from build123d import *

# Parameters (mm, degrees)
EXTRUDE_1_DEPTH     = 26
SKETCH_2_R          = 3.5
SKETCH_2_R_2        = 1.6
SKETCH_2_R_3        = 2
CUT_EXTRUDE_2_DEPTH = 155.518607294
CUT_EXTRUDE_5_DEPTH = 155.518607294
SKETCH_5_R          = 10.5
CUT_EXTRUDE_6_DEPTH = 1.6
CUT_EXTRUDE_START   = -1.6
SKETCH_6_R          = 10.5
CUT_EXTRUDE_7_DEPTH = 1.6
SKETCH_7_R          = 10.5
CUT_EXTRUDE_8_DEPTH = 1.6
SKETCH_8_R          = 10.5
CUT_EXTRUDE_9_DEPTH = 1.6


with BuildPart() as part:
    # 草图1 → 凸台-拉伸1 (new body)
    with BuildSketch(Plane(origin=(0, 0, 0), x_dir=(1, 0, 0), z_dir=(0, 1, 0))):
        with BuildLine():
            Line((0, 0), (0, 140))
            Line((0, 140), (5, 140))
            Line((5, 140), (5, 85))
            ThreePointArc((5, 85), (7.928932188, 77.928932188), (15, 75))
            Line((15, 75), (45, 75))
            ThreePointArc((45, 75), (52.071067812, 77.928932188), (55, 85))
            Line((55, 85), (55, 140))
            Line((55, 140), (60, 140))
            Line((60, 140), (60, 0))
            Line((60, 0), (55, 0))
            Line((55, 0), (55, 55))
            ThreePointArc((55, 55), (52.071067812, 62.071067812), (45, 65))
            Line((45, 65), (15, 65))
            ThreePointArc((15, 65), (7.928932188, 62.071067812), (5, 55))
            Line((5, 55), (5, 0))
            Line((5, 0), (0, 0))
        make_face()
    extrude(amount=EXTRUDE_1_DEPTH)

    # 草图2 → 切除-拉伸2 (cut, through all)
    with BuildSketch(Plane(origin=(60, 0, 0), x_dir=(0, 0, -1), z_dir=(1, 0, 0))):
        with Locations((128, 13)):
            Circle(SKETCH_2_R)
        with Locations((123, 18)):
            Circle(SKETCH_2_R_2)
        with Locations((133, 18)):
            Circle(SKETCH_2_R_2)
        with Locations((133, 8)):
            Circle(SKETCH_2_R_2)
        with Locations((123, 8)):
            Circle(SKETCH_2_R_2)
        with Locations((12, 13)):
            Circle(SKETCH_2_R)
        with Locations((7, 18)):
            Circle(SKETCH_2_R_2)
        with Locations((7, 8)):
            Circle(SKETCH_2_R_2)
        with Locations((17, 8)):
            Circle(SKETCH_2_R_2)
        with Locations((17, 18)):
            Circle(SKETCH_2_R_2)
        with Locations((28, 13)):
            Circle(SKETCH_2_R_3)
        with Locations((44, 13)):
            Circle(SKETCH_2_R_3)
        with Locations(Location((96, 13, 0), (0, 0, 180))):
            Circle(SKETCH_2_R_3)
        with Locations(Location((112, 13, 0), (0, 0, 180))):
            Circle(SKETCH_2_R_3)
    extrude(amount=-CUT_EXTRUDE_2_DEPTH, mode=Mode.SUBTRACT)

    # 草图3 → 切除-拉伸5 (cut, through all)
    with BuildSketch(Plane.ZY):
        with BuildLine():
            Line((-127, 26), (-140, 26))
            Line((-140, 26), (-140, 13))
            ThreePointArc((-140, 13), (-136.192388155, 22.192388155), (-127, 26))
        make_face()
        with BuildLine():
            ThreePointArc((-127, 0), (-136.192388155, 3.807611845), (-140, 13))
            Line((-140, 13), (-140, 0))
            Line((-140, 0), (-127, 0))
        make_face()
        with BuildLine():
            ThreePointArc((0, 13), (-3.807611845, 3.807611845), (-13, 0))
            Line((-13, 0), (0, 0))
            Line((0, 0), (0, 13))
        make_face()
        with BuildLine():
            Line((0, 26), (-13, 26))
            ThreePointArc((-13, 26), (-3.807611845, 22.192388155), (0, 13))
            Line((0, 13), (0, 26))
        make_face()
    extrude(amount=-CUT_EXTRUDE_5_DEPTH, mode=Mode.SUBTRACT)

    # 草图5 → 切除-拉伸6 (cut)
    with BuildSketch(Plane.ZY.offset(-55)):
        with Locations((-128, 13)):
            Circle(SKETCH_5_R)
    extrude(amount=-CUT_EXTRUDE_6_DEPTH, mode=Mode.SUBTRACT)

    # 草图6 → 切除-拉伸7 (cut)
    with BuildSketch(Plane(origin=(5, 0, 0), x_dir=(0, 0, -1), z_dir=(1, 0, 0)).offset(CUT_EXTRUDE_START)):
        with Locations(Location((128, 13, 0), (0, 0, 180))):
            Circle(SKETCH_6_R)
    extrude(amount=CUT_EXTRUDE_7_DEPTH, mode=Mode.SUBTRACT)

    # 草图7 → 切除-拉伸8 (cut)
    with BuildSketch(Plane.ZY.offset(-55)):
        with Locations((-12, 13)):
            Circle(SKETCH_7_R)
    extrude(amount=-CUT_EXTRUDE_8_DEPTH, mode=Mode.SUBTRACT)

    # 草图8 → 切除-拉伸9 (cut)
    with BuildSketch(Plane(origin=(5, 0, 0), x_dir=(0, 0, -1), z_dir=(1, 0, 0)).offset(CUT_EXTRUDE_START)):
        with Locations(Location((12, 13, 0), (0, 0, 180))):
            Circle(SKETCH_8_R)
    extrude(amount=CUT_EXTRUDE_9_DEPTH, mode=Mode.SUBTRACT)


solid = part.part
For this review, take the finished solid that the model builds, in its own axes (mm). A direction names the side the tool comes from. Give positions to 0.01 mm unless a question says otherwise; leave off trailing zeros. Loops run counter-clockwise (first coordinate to the right, second up) from the corner with the lowest first, then second, coordinate; pieces in that order, holes last. Notation, with made-up numbers: M 63.5,49.5 L 68.5,49.5 A31 cw 68.5,73.5 Z; hole C 81,74.5 d2. An arc over 180 degrees is marked long. Put each result on its own line as item: value. Start each with the question number.
(1) Add section C-C, the plane x = 17. Write out the cut boundary in (y, z), then the cut area to 3 significant figures.
(2) For pin 1 (8 mm diameter, centred on x = 13.5, y = 17.5, fed in from -Z); pin 2 (1.5 mm diameter, centred on x = 42, y = 7.5, fed in from -Z); pin 3 (8 mm diameter, centred on x = 14, z = -62.5, fed in from -Y); pin 4 (10 mm diameter, centred on x = 15, y = 20.5, fed in from +Z), all flat-tipped, find the tip position at first contact; note any pin that passes through.
(3) Machinability: for faces 3 (the flat face through (55, 13, -33)), 4 (the cylindrical face through (57.535, 13.601, -29.908)), 5 (the flat face through (60, 13, -71)), 6 (the cylindrical face through (7.85, 12.82, -78.01)), 7 (the cylindrical face through (55.8, 16.2, -2)), which of the approach directions +Z, -Z, +X, -X, +Y, -Y give a long, thin tool a straight path to every point of the face, cutting with its end or side? Answer none if there is none.
(4) Add section A-A, the plane z = -96. Write out the cut boundary in (x, y).
(5) Wall thickness on L1, parallel to Y at x = 1, z = -17; L2, parallel to X at y = 5.5, z = -115; L3, parallel to X at y = 16.75, z = -131: over which ranges is each line inside the solid? List them lowest first.
(6) Add section B-B, the plane z = -133. Give the number of separate pieces and of enclosed holes in the cut face, then the cut area to 3 significant figures.
(7) The part is to be moulded in two halves that separate along Y. For faces 1 (the cylindrical face through (52.15, 12.82, -61.99)), 2 (the flat face through (3.4, 13, -123)), say which applies: +Y half, -Y half, draft (parallel to the pull), parting line (faces both ways), or undercut.
Result:
1. outline: M 0,-75 L 26,-75 L 26,-65 L 0,-65 Z
1. area: 260 mm^2
2. pin 1: stops at z = -76.65
2. pin 2: stops at z = -75
2. pin 3: stops at y = 0
2. pin 4: stops at z = -63.66
3. face 3: +Z, +Y, -Y
3. face 4: +X, -X
3. face 5: +Z, -Z, +X, +Y, -Y
3. face 6: -Z, +Y, -Y
3. face 7: none
4. outline: M 0,0 L 5,0 L 5,11 L 0,11 Z; M 0,15 L 5,15 L 5,26 L 0,26 Z; M 55,0 L 60,0 L 60,11 L 55,11 Z; M 55,15 L 60,15 L 60,26 L 55,26 Z
5. L1: y = 0 to 6.4, 9.6 to 16.4, 19.6 to 26
5. L2: x = 0 to 5, 55 to 60
5. L3: x = 0 to 3.4, 56.6 to 60
6. separate pieces: 6
6. enclosed holes: 0
6. area: 128 mm^2
7. face 1: draft
7. face 2: undercut
